Input: dimensioned drawing with shaded views. Units: mm. Origin: part minimum x, y, z. A direction names the side the tool comes from. Give positions to 0.01 mm unless a question says otherwise; leave off trailing zeros. Order: outer loops, then holes, each group sorted by start corner. A loop starts at its lowest first (then second) coordinate and runs counter-clockwise, first axis right, second up. Notation, with made-up numbers: (40.25, -1) -> (60.25, -1) arc R34 cw to (60.25, 36) -> close; hole circle Ø2 at (78, 71). An arc over 180 degrees is marked (long way). One line per question, with ' | ' between items. Start each with the question number.
(1) Section D-D (y = 2). Return loops of the section in (x, z) (1 decimal).
(2) Section B-B (z = 14). Return loops of the section in (x, y).
(3) First-contact query: pin 1 Ø1 at (y, z) = (4.5, 19) entering from -X; pin 2 Ø2.5 at (x, z) = (1, 14) entering from +Y; pin 3 Ø1 at (x, y) = (1.5, 9.5) entering from +Z. Flat tips, straight axial feed; report the tip coordinate or a pass-through.
(4) Mould query, pull axis Y, two halves, no side actions, for the marked faces 4, 5, 6 and 7. Classes: +Y half, -Y half, draft (parallel to the pull), parting line (faces both ways), or undercut.
(5) Section C-C (x = 4.5). State how many separate pieces and enclosed holes the cut face has.
(6) Set-up query: the marked faces 1, 2 and 3. Return all of +Z, -Z, +X, -X, +Y, -Y with unobstructed straight access to the full face (end or side cutting, diameter ignored); none if empty.
(7) Section A-A (y = 6.35). Return loops of the section in (x, z) (1 decimal), then the cut area to 3 significant figures.
(8) Ray query, L1, parallel to Z at x = 7.1, y = 6.35; L2, parallel to X at y = 7.75, z = 20.5; L3, parallel to Z at x = 4, y = 12.7 (1 decimal). Return the intervals inside material, ascending.
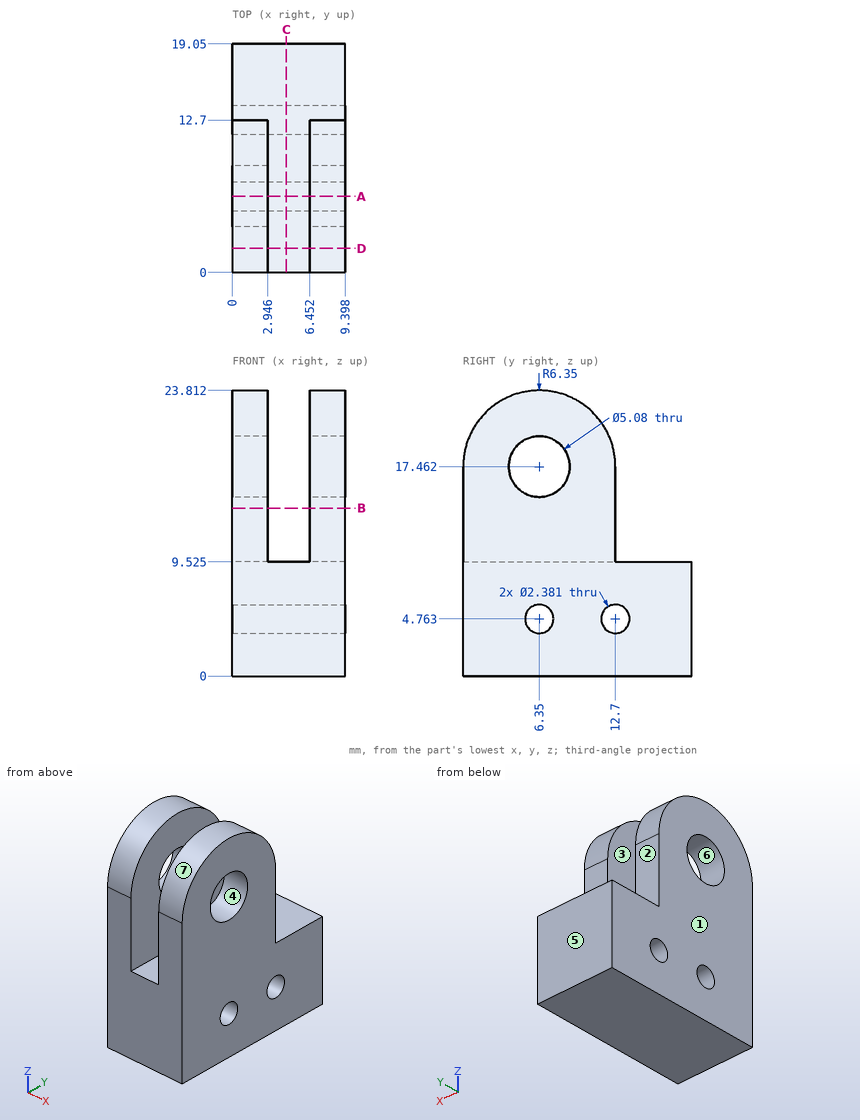
Response:
1) outline: (0, 0) -> (9.4, 0) -> (9.4, 22.1) -> (6.5, 22.1) -> (6.5, 9.5) -> (2.9, 9.5) -> (2.9, 22.1) -> (0, 22.1) -> close
2) outline: (0, 0) -> (2.95, 0) -> (2.95, 12.7) -> (0, 12.7) -> close; (6.45, 0) -> (9.4, 0) -> (9.4, 12.7) -> (6.45, 12.7) -> close
3) pin 1: stops at x = 0 | pin 2: stops at y = 12.7 | pin 3: stops at z = 23.23
4) face 4: undercut | face 5: +Y half | face 6: undercut | face 7: parting line
5) separate pieces: 1 | enclosed holes: 2
6) face 1: +Z, -Z, -X, +Y, -Y | face 2: +Z, +X, -X, +Y | face 3: +Z, +Y, -Y
7) outline: (0, 0) -> (9.4, 0) -> (9.4, 3.6) -> (0, 3.6) -> close; (0, 6) -> (9.4, 6) -> (9.4, 14.9) -> (6.5, 14.9) -> (6.5, 9.5) -> (2.9, 9.5) -> (2.9, 14.9) -> (0, 14.9) -> close; (0, 20) -> (2.9, 20) -> (2.9, 23.8) -> (0, 23.8) -> close; (6.5, 20) -> (9.4, 20) -> (9.4, 23.8) -> (6.5, 23.8) -> close | area: 121 mm^2
8) L1: z = 0 to 3.57, 5.95 to 14.92, 20 to 23.81 | L2: x = 0 to 2.95, 6.45 to 9.4 | L3: z = 0 to 3.6, 6 to 9.5
